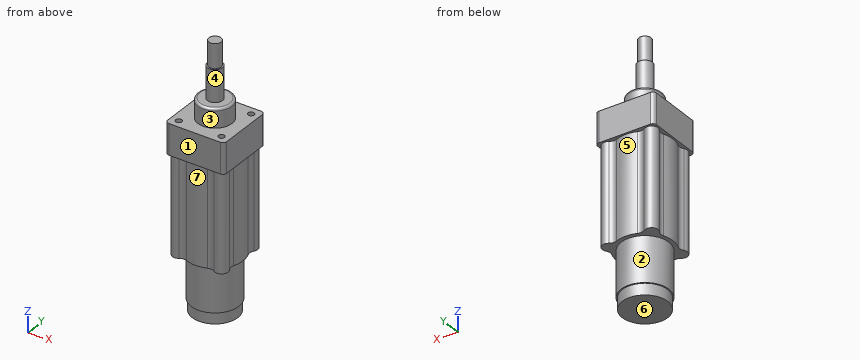
from build123d import *

# Parameters (mm, degrees)
SALIENTE_EXTRUIR1_DEPTH = 40.5
CROQUIS2_R              = 36.886156795
SALIENTE_EXTRUIR2_DEPTH = 170.5
CROQUIS3_R              = 31.5
SALIENTE_EXTRUIR3_DEPTH = 230.5
CROQUIS4_R              = 30
SALIENTE_EXTRUIR4_DEPTH = 15
CROQUIS5_R              = 8.5
SALIENTE_EXTRUIR5_DEPTH = 170.5
REDONDEO2_R             = 10
REDONDEO3_R             = 10
REDONDEO4_R             = 10
REDONDEO5_R             = 10
CROQUIS6_R              = 4
CORTAR_EXTRUIR1_DEPTH   = 17.5
CROQUIS7_R              = 22.5
SALIENTE_EXTRUIR7_DEPTH = 25
REDONDEO6_R             = 3
CROQUIS8_R              = 10
SALIENTE_EXTRUIR8_DEPTH = 42
CROQUIS9_R              = 8
SALIENTE_EXTRUIR9_DEPTH = 32


with BuildPart() as part:
    # Croquis1 → Saliente-Extruir1 (new body)
    with BuildSketch(Plane.XY):
        with BuildLine():
            Line((-34, -39), (34, -39))
            ThreePointArc((34, -39), (37.535533906, -37.535533906), (39, -34))
            Line((39, -34), (39, 34))
            ThreePointArc((39, 34), (37.535533906, 37.535533906), (34, 39))
            Line((34, 39), (-34, 39))
            ThreePointArc((-34, 39), (-37.535533906, 37.535533906), (-39, 34))
            Line((-39, 34), (-39, -34))
            ThreePointArc((-39, -34), (-37.535533906, -37.535533906), (-34, -39))
        make_face()
    extrude(amount=-SALIENTE_EXTRUIR1_DEPTH)

    # Croquis2 → Saliente-Extruir2 (add)
    with BuildSketch(Plane.XY):
        Circle(CROQUIS2_R)
    extrude(amount=-SALIENTE_EXTRUIR2_DEPTH)

    # Croquis3 → Saliente-Extruir3 (add)
    with BuildSketch(Plane.XY):
        Circle(CROQUIS3_R)
    extrude(amount=-SALIENTE_EXTRUIR3_DEPTH)

    # Croquis4 → Saliente-Extruir4 (add)
    with BuildSketch(Plane(origin=(0, 0, -230.5), x_dir=(-1, 0, 0), z_dir=(0, 0, -1))):
        Circle(CROQUIS4_R)
    extrude(amount=SALIENTE_EXTRUIR4_DEPTH)

    # Croquis5 → Saliente-Extruir5 (add)
    with BuildSketch(Plane.XY):
        with Locations((28.25, 28.25)):
            Circle(CROQUIS5_R)
        with Locations((28.25, -28.25)):
            Circle(CROQUIS5_R)
        with Locations((-28.25, -28.25)):
            Circle(CROQUIS5_R)
        with Locations((-28.25, 28.25)):
            Circle(CROQUIS5_R)
    extrude(amount=-SALIENTE_EXTRUIR5_DEPTH)

    # Redondeo2
    redondeo2_edges = [part.edges().sort_by_distance(p)[0] for p in [
        (20.168422903, 30.884029541, -105.5),
        (-20.168422903, 30.884029541, -105.5),
    ]]
    fillet(redondeo2_edges, radius=REDONDEO2_R)

    # Redondeo3
    redondeo3_edges = [part.edges().sort_by_distance(p)[0] for p in [
        (-30.884029541, -20.168422903, -105.5),
        (-30.884029541, 20.168422903, -105.5),
    ]]
    fillet(redondeo3_edges, radius=REDONDEO3_R)

    # Redondeo4
    redondeo4_edges = [part.edges().sort_by_distance(p)[0] for p in [
        (20.168422903, -30.884029541, -105.5),
        (-20.168422903, -30.884029541, -105.5),
    ]]
    fillet(redondeo4_edges, radius=REDONDEO4_R)

    # Redondeo5
    redondeo5_edges = [part.edges().sort_by_distance(p)[0] for p in [
        (30.884029541, 20.168422903, -105.5),
        (30.884029541, -20.168422903, -105.5),
    ]]
    fillet(redondeo5_edges, radius=REDONDEO5_R)

    # Croquis6 → Cortar-Extruir1 (cut)
    with BuildSketch(Plane.XY):
        with Locations((28.25, 28.25)):
            Circle(CROQUIS6_R)
        with Locations((-28.25, 28.25)):
            Circle(CROQUIS6_R)
        with Locations((28.25, -28.25)):
            Circle(CROQUIS6_R)
        with Locations((-28.25, -28.25)):
            Circle(CROQUIS6_R)
    extrude(amount=-CORTAR_EXTRUIR1_DEPTH, mode=Mode.SUBTRACT)

    # Croquis7 → Saliente-Extruir7 (add)
    with BuildSketch(Plane.XY):
        Circle(CROQUIS7_R)
    extrude(amount=SALIENTE_EXTRUIR7_DEPTH)

    # Redondeo6
    redondeo6_edges = [part.edges().sort_by_distance(p)[0] for p in [
        (-22.5, 0, 25),
    ]]
    fillet(redondeo6_edges, radius=REDONDEO6_R)

    # Croquis8 → Saliente-Extruir8 (add)
    with BuildSketch(Plane.XY.offset(25)):
        Circle(CROQUIS8_R)
    extrude(amount=SALIENTE_EXTRUIR8_DEPTH)

    # Croquis9 → Saliente-Extruir9 (add)
    with BuildSketch(Plane.XY.offset(67)):
        Circle(CROQUIS9_R)
    extrude(amount=SALIENTE_EXTRUIR9_DEPTH)


solid = part.part
The model under review builds one solid part; all positions refer to its coordinate system, in mm. Face numbers are marked on the shaded views. A direction names the side the tool comes from. Coordinates: 2 decimals unless noted, no trailing zeros. Use a Markdown table: item, result. Add a question column.
1. Machinability: for the marked faces 1, 2 and 3, which of the approach directions +Z, -Z, +X, -X, +Y, -Y give a long, thin tool a straight path to every point of the face, cutting with its end or side? Answer none if there is none.
2. Draft analysis for pull direction X (two halves, no side actions). For the marked faces 4, 5, 6 and 7, state which applies: pulls with the +X half, pulls with the -X half, needs draft (parallel to the pull), parting line crosses it, or undercut.
3. Clearance check with flat-ended pins moving along their axes: pin 1 Ø2 at (y, z) = (-5, 33.5) entering from -X; pin 2 Ø3 at (y, z) = (-27.5, -108) entering from -X; pin 3 Ø6.5 at (x, y) = (-27.5, 30) entering from +Z. State where each tip first meets the part, or that it passes through.
4. To check wall thickness, follow line 1 (X direction, y = -28, z = -9); line 2 (Y direction, x = 28.25, z = -7); line 3 (Z direction, x = -10.5, y = 17). State the ranges of each line that lie inside material, in increasing order.
Returned:
| question | item | result |
|---|---|---|
| 1 | face 1 | +Z, -Z, +X, -X, -Y |
| 1 | face 2 | -Z |
| 1 | face 3 | +Z |
| 2 | face 4 | parting line crosses it |
| 2 | face 5 | undercut |
| 2 | face 6 | needs draft |
| 2 | face 7 | undercut |
| 3 | pin 1 | stops at x = -9.17 |
| 3 | pin 2 | stops at x = -36.75 |
| 3 | pin 3 | stops at z = 0 |
| 4 | line 1 | x = -39 to -32.24, -24.26 to 24.26, 32.24 to 39 |
| 4 | line 2 | y = -39 to -32.25, -24.25 to 24.25, 32.25 to 39 |
| 4 | line 3 | z = -245.5 to 24.96 |
